from build123d import *

# Parameters (mm, degrees)
PAD002_DEPTH            = 30
SKETCH005_R             = 1.75
POCKET009_DEPTH         = 33.001
FILLET009_R             = 9
FILLET010_R             = 1
BODY001_ROLL_ANGLE      = -90
BODY001_PLACEMENT_ANGLE = 90


with BuildPart() as part:
    # Sketch004 (on XY_Plane001 of Origin002) → Pad002 (new body)
    with BuildSketch(Plane.XY):
        with BuildLine():
            Line((0, 25), (-3, 25))
            Line((-3, 25), (-3, 0))
            ThreePointArc((-26.999998, 0.006802), (-15.003401, -12), (-3, 0))
            Line((-29.999998, 0.006802), (-26.999998, 0.006802))
            ThreePointArc((-29.999998, 0.006802), (-15.003401, -15), (0, 0))
            Line((0, 0), (0, 25))
        make_face()
    extrude(amount=PAD002_DEPTH)

    # Sketch005 (on Face2 of Pad002) → Pocket009 (cut, through all)
    with BuildSketch(Plane(origin=(-33, 0, 0), x_dir=(0, -1, 0), z_dir=(-1, 0, 0))):
        with Locations((-12.5, 7.5)):
            Circle(SKETCH005_R)
        with Locations((-12.5, 22.5)):
            Circle(SKETCH005_R)
    extrude(amount=-POCKET009_DEPTH, mode=Mode.SUBTRACT)

    # Fillet009
    fillet009_edges = [part.edges().sort_by_distance(p)[0] for p in [
        (-28.499998, 0.006802, 30),
        (-28.499998, 0.006802, 0),
    ]]
    fillet(fillet009_edges, radius=FILLET009_R)

    # Fillet010
    fillet010_edges = [part.edges().sort_by_distance(p)[0] for p in [
        (-1.5, 25, 30),
        (-1.5, 25, 0),
    ]]
    fillet(fillet010_edges, radius=FILLET010_R)


with BuildPart() as part_1:
    # Body001 roll: moved
    add(part.part.rotate(Axis((0, 0, 0), (1, 0, 0)), BODY001_ROLL_ANGLE))


with BuildPart() as part_2:
    # Body001 placement: moved
    add(part_1.part.moved(Location((15, -17.1, 25))).rotate(Axis((15, -17.1, 25), (0, 0, 1)), BODY001_PLACEMENT_ANGLE))


solid = part_2.part
Can you work these out from the model? Positions are in its coordinate system, mm. A direction names the side the tool comes from. Give positions to 0.01 mm unless a question says otherwise; leave off trailing zeros. Loops run counter-clockwise (first coordinate to the right, second up) from the corner with the lowest first, then second, coordinate; pieces in that order, holes last. Notation, with made-up numbers: (78, 5.25) -> (126, 5.25) arc R13 ccw to (126, 23.25) -> close; hole circle Ø6 at (52.5, -4.5). An arc over 180 degrees is marked (long way). Write item = value, one per line.
1) Suppose I cut it at A-A on z = 27.5. Write out the boundary of the cut face in (x, y).
Check result:
outline = (-15, -20.36) -> (15, -20.36) -> (15, -17.31) -> (-15, -17.31) -> close; (-12.23, -46.89) -> (12.23, -46.89) -> (12.23, -43.84) -> (-12.23, -43.84) -> close
2) Suppose I cut it at D-D on y = -42. Write out the boundary of the cut face in (x, z).
Check result:
outline = (-15, 33.99) arc R9 ccw to (-14.72, 31.78) -> (14.72, 31.78) arc R9 ccw to (15, 33.99) -> (15, 36.27) -> (-15, 36.27) -> close
3) Suppose I cut it at C-C on x = -0.5. Write out the boundary of the cut face in (y, z), then the cut area to 3 significant figures.
Check result:
outline = (-47.1, 24.99) -> (-44.1, 24.99) arc R12 cw to (-20.1, 25) -> (-20.1, 0) -> (-17.1, 0) -> (-17.1, 25) arc R15 ccw to start
area = 202 mm2
4) For faces 4 (the cylindrical face through (12.434, -45.091, 27.7)), 5 (the cylindrical face through (-12.434, -45.091, 27.7)), 6 (the flat face through (0, -20.1, 12)), which set-ups out of +Z, -Z, +X, -X, +Y, -Y let a thin tool reach every point of the face, with its end or its side?
Check result:
face_4 = -Z, +X, -Y
face_5 = -Z, -X, -Y
face_6 = -Z, +X, -X, -Y
5) Suppose I cut it at B-B on x = -7.5. Write out the boundary of the cut face in (y, z).
Check result:
outline = (-47.1, 25.12) -> (-44.1, 25.12) arc R12 cw to (-20.1, 25) -> (-20.1, 14.25) -> (-17.1, 14.25) -> (-17.1, 25) arc R15 ccw to start; (-20.1, 0) -> (-17.1, 0) -> (-17.1, 10.75) -> (-20.1, 10.75) -> close
6) Will these pins go through, and if not, where does the flat tip stop? pin 1 (3 mm diameter, centred on x = 3.5, y = -26.5, fed in from +Z); pin 2 (2 mm diameter, centred on x = -3, z = 21, fed in from -Y); pin 3 (10 mm diameter, centred on y = -29, z = 27, fed in from -X); pin 4 (0.9 mm diameter, centred on x = 3, y = -46, fed in from -Z).
Check result:
pin_1 = 39.43
pin_2 = -20.1
pin_3 = through
pin_4 = 24.99
7) I need wall thicknesses on L1, parallel to X at y = -17.9, z = 12.5; L2, parallel to Y at x = 10, z = 21.5; L3, parallel to Y at x = -3, z = 34.5. Which ranges of each line are inside material? Lowest first, please. Write a range as from..to.
Check result:
L1 = -15..-9.25, -5.75..5.75, 9.25..15
L2 = -20.1..-17.1
L3 = -43.71..-39.43, -24.77..-20.49
8) Thinking about a two-plate mould opening in X: for faces 1 (the flat face through (-15, -19.7, 26.2)), 2 (the cylindrical face through (9.05, -18.62, 13.31)), 3 (the cylindrical face through (14.715, -18.621, 0.301)), which applies, released by +X, released by -X, zero draft, split by the parting line, or undercut?
Check result:
face_1 = released by -X
face_2 = undercut
face_3 = released by +X
